Design review of the part built by this model. Coordinates are the model's own, in mm. Face numbers are marked on the shaded views. Give positions to 0.01 mm unless a question says otherwise; leave off trailing zeros. Order: outer loops, then holes, each group sorted by start corner. A loop starts at its lowest first (then second) coordinate and runs counter-clockwise, first axis right, second up. Notation, with made-up numbers: (28.5, 46.25) -> (68.5, 46.25) arc R19 ccw to (68.5, 65.25) -> close; hole circle Ø7 at (-34, 29). An arc over 180 degrees is marked (long way). One line per item, written item: value.
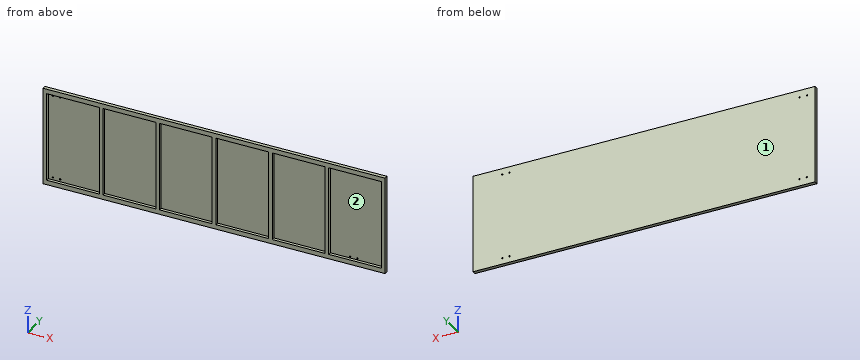
from build123d import *

# Parameters (mm, degrees)
F0_W     = 244.856
F0_H     = 414.782
F1_DEPTH = 17.018
F2_DEPTH = 2.54
F4_D     = 6.35
F4_DEPTH = 2.54
F4_TIP   = 1.9077324654


# Not quite as in the source:
# - a feature names something its author has since deleted; it is built from what else it names


with BuildPart() as f1:
    # F0 (on Front) → F1 (new body)
    with BuildSketch(Plane.XZ):
        Polygon((350.52, 228.6), (139.7, 228.6), (105.41, 228.6), (-139.7, 228.6), (-139.7, -228.6), (105.41, -228.6), (139.7, -228.6), (350.52, -228.6), (384.81, -228.6), (595.63, -228.6), (629.92, -228.6), (840.74, -228.6), (875.03, -228.6), (1085.85, -228.6), (1120.14, -228.6), (1365.25, -228.6), (1450.34, -228.6), (1450.34, 228.6), (1365.25, 228.6), (1120.14, 228.6), (1085.85, 228.6), (875.03, 228.6), (840.74, 228.6), (629.92, 228.6), (595.63, 228.6), (384.81, 228.6), align=None)
        Rectangle(F0_W, F0_H, mode=Mode.SUBTRACT)
        with Locations((262.128, 0)):
            Rectangle(F0_W, F0_H, mode=Mode.SUBTRACT)
        Polygon((629.92, 207.391), (646.684, 207.391), (646.684, -207.391), (629.92, -207.391), (401.828, -207.391), (401.828, 207.391), align=None, mode=Mode.SUBTRACT)
        Polygon((875.03, 207.391), (908.812, 207.391), (908.812, -207.391), (875.03, -207.391), (663.956, -207.391), (663.956, 207.391), align=None, mode=Mode.SUBTRACT)
        Polygon((1120.14, 207.391), (1170.94, 207.391), (1170.94, -207.391), (1120.14, -207.391), (926.084, -207.391), (926.084, 207.391), align=None, mode=Mode.SUBTRACT)
        with Locations((1310.64, 0)):
            Rectangle(F0_W, F0_H, mode=Mode.SUBTRACT)
    extrude(amount=F1_DEPTH)

    # F0 (on Front) → F2 (join)
    with BuildSketch(Plane.XZ):
        Polygon((350.52, 228.6), (139.7, 228.6), (105.41, 228.6), (-139.7, 228.6), (-139.7, -228.6), (105.41, -228.6), (139.7, -228.6), (350.52, -228.6), (384.81, -228.6), (595.63, -228.6), (629.92, -228.6), (840.74, -228.6), (875.03, -228.6), (1085.85, -228.6), (1120.14, -228.6), (1365.25, -228.6), (1450.34, -228.6), (1450.34, 228.6), (1365.25, 228.6), (1120.14, 228.6), (1085.85, 228.6), (875.03, 228.6), (840.74, 228.6), (629.92, 228.6), (595.63, 228.6), (384.81, 228.6), align=None)
        Rectangle(F0_W, F0_H, mode=Mode.SUBTRACT)
        with Locations((262.128, 0)):
            Rectangle(F0_W, F0_H, mode=Mode.SUBTRACT)
        Polygon((629.92, 207.391), (646.684, 207.391), (646.684, -207.391), (629.92, -207.391), (401.828, -207.391), (401.828, 207.391), align=None, mode=Mode.SUBTRACT)
        Polygon((875.03, 207.391), (908.812, 207.391), (908.812, -207.391), (875.03, -207.391), (663.956, -207.391), (663.956, 207.391), align=None, mode=Mode.SUBTRACT)
        Polygon((1120.14, 207.391), (1170.94, 207.391), (1170.94, -207.391), (1120.14, -207.391), (926.084, -207.391), (926.084, 207.391), align=None, mode=Mode.SUBTRACT)
        with Locations((1310.64, 0)):
            Rectangle(F0_W, F0_H, mode=Mode.SUBTRACT)
        Rectangle(F0_W, F0_H)
        with Locations((262.128, 0)):
            Rectangle(F0_W, F0_H)
        Polygon((646.684, -207.391), (646.684, 207.391), (629.92, 207.391), (401.828, 207.391), (401.828, -207.391), (629.92, -207.391), align=None)
        Polygon((908.812, -207.391), (908.812, 207.391), (875.03, 207.391), (663.956, 207.391), (663.956, -207.391), (875.03, -207.391), align=None)
        Polygon((1170.94, -207.391), (1170.94, 207.391), (1120.14, 207.391), (926.084, 207.391), (926.084, -207.391), (1120.14, -207.391), align=None)
        with Locations((1310.64, 0)):
            Rectangle(F0_W, F0_H)
    extrude(amount=F2_DEPTH)

    # F4
    with Locations(Plane(origin=(0, 0, 0), x_dir=(-1, 0, 0), z_dir=(0, 1, 0))):
        with Locations((-1314.45, 200.061827898), (-1280.31875, 200.061827898), (67.4624, 195.9268003702), (101.6, 195.9268003702), (-1314.45, -200.061827898), (-1280.31875, -200.061827898), (67.4624, -195.9268003702), (101.6, -195.9268003702)):
            Hole(F4_D / 2, depth=F4_DEPTH)
            with Locations((0, 0, -(F4_DEPTH + F4_TIP / 2))):  # 118° drill point
                Cone(0, F4_D / 2, F4_TIP, mode=Mode.SUBTRACT)


solid = f1.part
Item 1: Draft analysis for pull direction Z (two halves, no side actions). For the marked faces 1 and 2, state which applies: pulls with the +Z half, pulls with the -Z half, needs draft (parallel to the pull), parting line crosses it, or undercut.
Returned:
face 1: needs draft
face 2: undercut
Item 2: Add section C-C on z = -143.5. Give the boundary of the cut face in (x, y), plus the area to 3 significant figures.
Returned:
outline: (-139.7, -17.02) -> (-122.43, -17.02) -> (-122.43, -2.54) -> (122.43, -2.54) -> (122.43, -17.02) -> (139.7, -17.02) -> (139.7, -2.54) -> (384.56, -2.54) -> (384.56, -17.02) -> (401.83, -17.02) -> (401.83, -2.54) -> (646.68, -2.54) -> (646.68, -17.02) -> (663.96, -17.02) -> (663.96, -2.54) -> (908.81, -2.54) -> (908.81, -17.02) -> (926.08, -17.02) -> (926.08, -2.54) -> (1170.94, -2.54) -> (1170.94, -17.02) -> (1188.21, -17.02) -> (1188.21, -2.54) -> (1433.07, -2.54) -> (1433.07, -17.02) -> (1450.34, -17.02) -> (1450.34, 0) -> (-139.7, 0) -> close
area: 5,790 mm²
Item 3: Add section A-A on x = 75. Give the boundary of the cut face in (y, z).
Returned:
outline: (-17.02, -228.6) -> (0, -228.6) -> (0, 228.6) -> (-17.02, 228.6) -> (-17.02, 207.39) -> (-2.54, 207.39) -> (-2.54, -207.39) -> (-17.02, -207.39) -> close
Item 4: Add section B-B on y = -10.25. Give the boundary of the cut face in (x, z).
Returned:
outline: (-139.7, -228.6) -> (1450.34, -228.6) -> (1450.34, 228.6) -> (-139.7, 228.6) -> close; hole (-122.43, -207.39) -> (122.43, -207.39) -> (122.43, 207.39) -> (-122.43, 207.39) -> close; hole (139.7, -207.39) -> (384.56, -207.39) -> (384.56, 207.39) -> (139.7, 207.39) -> close; hole (401.83, -207.39) -> (646.68, -207.39) -> (646.68, 207.39) -> (401.83, 207.39) -> close; hole (663.96, -207.39) -> (908.81, -207.39) -> (908.81, 207.39) -> (663.96, 207.39) -> close; hole (926.08, -207.39) -> (1170.94, -207.39) -> (1170.94, 207.39) -> (926.08, 207.39) -> close; hole (1188.21, -207.39) -> (1433.07, -207.39) -> (1433.07, 207.39) -> (1188.21, 207.39) -> close
Item 5: Clearance check with a flat-ended pin moving along its axis: P1, Ø3, axis at x = 538, z = 43, coming from the -Y side. State where the tip first meets the part, or that it passes through.
Returned:
P1: y = -2.54
Item 6: To check wall thickness, follow line 1 along Z through (x, y) = (942, -6.25); line 2 along Z through (x, y) = (-101.6, -0.8); line 3 along Y through (x, z) = (214.5, -28). State the ranges of each line that lie inside material, in increasing order. Write a range as from..to.
Returned:
line 1: -228.6..-207.39, 207.39..228.6
line 2: -228.6..-199.1, -192.75..192.75, 199.1..228.6
line 3: -2.54..0
